Geometry check sheet. Reference: the model listing, model coordinates, mm. Face numbers are marked on the shaded views. A direction names the side the tool comes from. Coordinates: 2 decimals unless noted, no trailing zeros. Order: outer loops, then holes, each group sorted by start corner. A loop starts at its lowest first (then second) coordinate and runs counter-clockwise, first axis right, second up. Notation, with made-up numbers: M -22.75,-4 L 32.25,-4 A19 ccw 32.25,30 Z; hole C 11,76.25 d10. An arc over 180 degrees is marked long. One line per item, written item: value. Start each with the question number.
1) Thickness scan on L1, parallel to Y at x = 48, z = 32.5; L2, parallel to X at y = 26.5, z = 16; L3, parallel to X at y = -52.5, z = 1.05. Record the ranges inside material, lowest first. Write a range as from..to.
2) Sectioned sample at A-A, the plane y = 0. Enter the section's corners in (x, z).
3) Go/stop test with flat-tipped pins: P1, Ø1.3, axis at x = -39, y = -61.5, coming from the -Z side; P2, Ø1, axis at x = 58.5, y = -14.5, coming from the +Z side; P3, Ø10, axis at x = -46, y = -20, coming from the +Z side; P4, Ø1, axis at y = -61, z = 108, coming from the -X side. Record where each tip stops, or that it passes through.
4) Sectioned sample at B-B, the plane z = 23.5. Enter the section's corners in (x, y).
5) Sectioned sample at C-C, the plane x = -11.5. Enter the section's corners in (y, z), then the cut area to 3 significant figures.
6) Access from +Z, -Z, +X, -X, +Y, -Y to the whole of each face (thin tool, end or side, straight path). Record for the marked faces 1 and 2.
7) Draft check along Y on the marked faces 3, 4 and 5. Enter one of: pulls with the +Y half, pulls with the -Y half, needs draft (parallel to the pull), parting line crosses it, or undercut.
```python
from build123d import *

# Parameters (mm, degrees)
F0_W     = 120
F0_H     = 120
F0_R     = 57.5
F1_DEPTH = 2
F2_DEPTH = 120
F3_D     = 3
F5_DEPTH = 122.001
F6_W     = 20
F6_H     = 4
F7_DEPTH = 124.001
F8_W     = 2
F8_H     = 120
F9_DEPTH = 30
F10_R    = 5


with BuildPart() as f1:
    # F0 (on Top) → F1 (new body)
    with BuildSketch(Plane.XY):
        Rectangle(F0_W, F0_H)
        Circle(F0_R, mode=Mode.SUBTRACT)
    extrude(amount=F1_DEPTH)

    # F0 (on Top) → F2 (join)
    with BuildSketch(Plane.XY):
        Polygon((60, -62), (60, -60), (-60, -60), (-60, 60), (60, 60), (60, 62), (-62, 62), (-62, -62), align=None)
    extrude(amount=F2_DEPTH)

    # F3 (through all)
    with Locations(Plane(origin=(0, 0, 0), x_dir=(1, 0, 0), z_dir=(0, 0, -1))):
        with Locations((52.5, 52.5), (52.5, -52.5), (-52.5, -52.5), (-52.5, 52.5)):
            Hole(F3_D / 2)

    # F4 (on face) → F5 (cut, through all)
    with BuildSketch(Plane(origin=(-62, 0, 0), x_dir=(0, -1, 0), z_dir=(-1, 0, 0))):
        with BuildLine():
            Line((62, 120), (-62, 120))
            ThreePointArc((-62, 120), (0, 60), (62, 120))
        make_face()
    extrude(amount=-F5_DEPTH, mode=Mode.SUBTRACT)

    # F6 (on face) → F7 (cut, through all)
    with BuildSketch(Plane.XZ.offset(62)):
        with Locations((-42, 108)):
            Rectangle(F6_W, F6_H)
    extrude(amount=-F7_DEPTH, mode=Mode.SUBTRACT)

    # F8 (on face) → F9 (join)
    with BuildSketch(Plane.XY.offset(2)):
        with Locations((59, 0)):
            Rectangle(F8_W, F8_H)
    extrude(amount=F9_DEPTH)

    # F10
    f10_edges = [f1.edges().sort_by_distance(p)[0] for p in [
        (59, 60, 32),
        (59, -60, 32),
        (-60, -60, 54.140525),
        (-62, -62, 60),
        (-62, 62, 60),
        (-60, 60, 54.140525),
    ]]
    fillet(f10_edges, radius=F10_R)


solid = f1.part
```
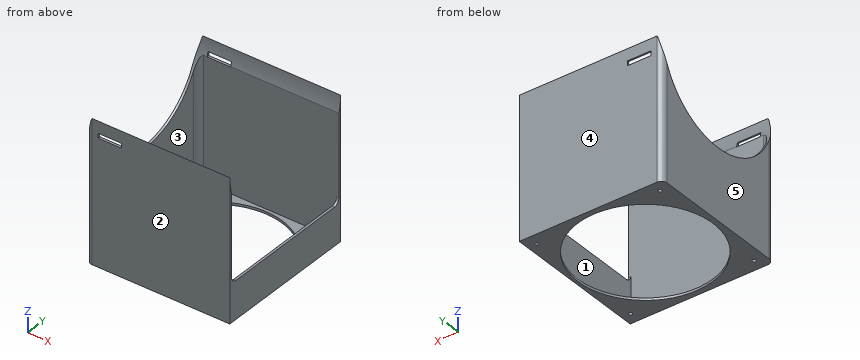
Final values:
1. L1: y = -62..-60, 60..62
1. L2: x = -62..-60, 58..60
1. L3: x = -62..-54, -51..-23.45, 23.45..51, 54..60
2. outline: M -62,0 L -57.5,0 L -57.5,2 L -60,2 L -60,60 L -62,60 Z; M 57.5,0 L 60,0 L 60,32 L 58,32 L 58,2 L 57.5,2 Z
3. P1: stops at z = 0
3. P2: stops at z = 32
3. P3: passes through
3. P4: stops at x = -60.57
4. outline: M -62,-57 A5 ccw -57,-62 L 60,-62 L 60,62 L -57,62 A5 ccw -62,57 Z; hole M -60,-55 A5 ccw -55,-60 L 58,-60 L 58,60 L -55,60 A5 ccw -60,55 Z
5. outline: M -62,0 L -56.34,0 L -56.34,2 L -60,2 L -60,106.28 A62.03 cw -62,120 Z; M 56.34,0 L 62,0 L 62,120 A62.03 cw 60,106.28 L 60,2 L 56.34,2 Z
5. area: 460 mm^2
6. face 1: +Z
6. face 2: +Z, -Z, +X, -X, -Y
7. face 3: undercut
7. face 4: pulls with the +Y half
7. face 5: needs draft
